Check sheet for the drawn part. Datum: minimum x, y, z corner. Units: mm. A direction names the side the tool comes from. Give positions to 0.01 mm unless a question says otherwise; leave off trailing zeros. Order: outer loops, then holes, each group sorted by start corner. A loop starts at its lowest first (then second) coordinate and runs counter-clockwise, first axis right, second up.
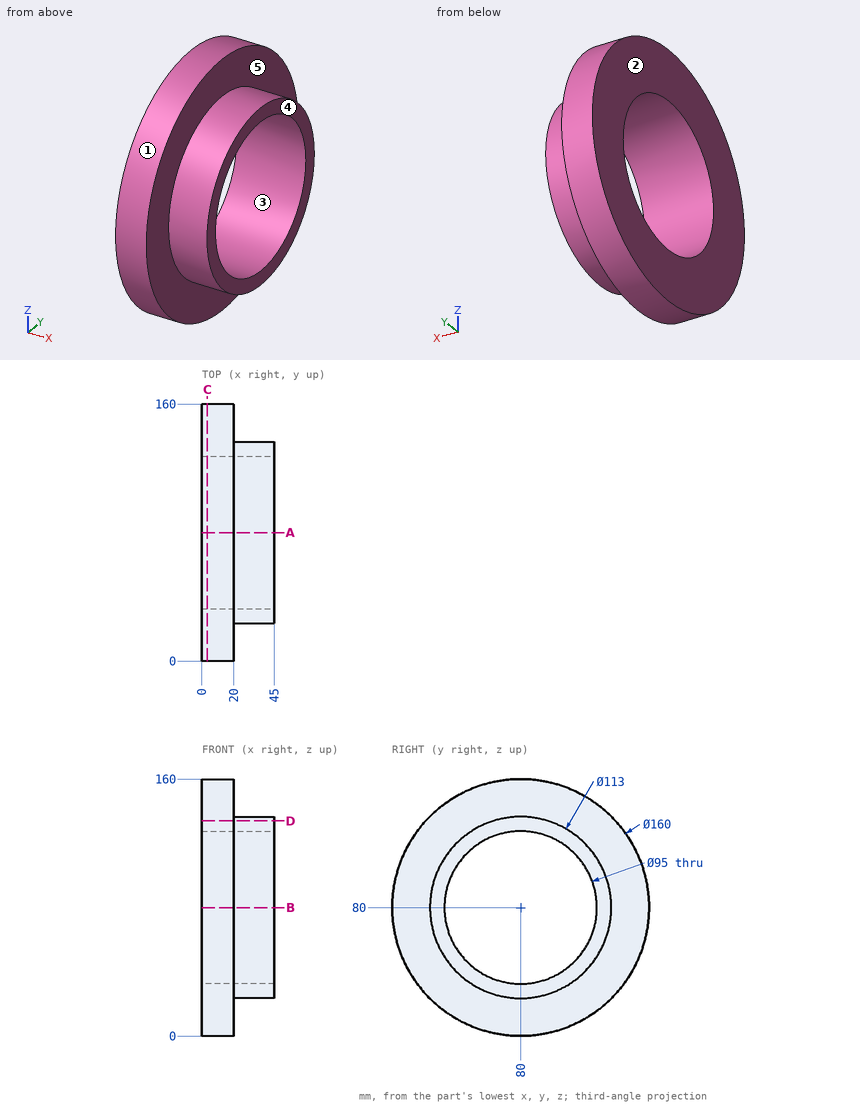
Item 1: Sectioned sample at D-D (z = 134). Enter the section's corners in (x, y), and give its area (3 significant figures).
Reported:
outline: (0, 20.97) - (20, 20.97) - (20, 63.38) - (45, 63.38) - (45, 96.62) - (20, 96.62) - (20, 139.03) - (0, 139.03) - close
area: 3,190 mm2
Item 2: Gauge pin test, flat ends, axial feed: pin 1 (4 mm diameter, centred on x = 33.5, z = 51.5, fed in from +Y); pin 2 (12 mm diameter, centred on y = 129.5, z = 111, fed in from +X); pin 3 (8 mm diameter, centred on x = 30, y = 90.5, fed in from +Z); pin 4 (5 mm diameter, centred on x = 15, y = 63, fed in from -Z). Record the tip position at first contact, or that the pin passes through.
Reported:
pin 1: stops at y = 129.9
pin 2: stops at x = 45
pin 3: stops at z = 136.12
pin 4: stops at z = 1.33
Item 3: Scan lines: L1, parallel to Y at x = 12.5, z = 80; L2, parallel to Y at x = 26, z = 80; L3, parallel to X at y = 57.5, z = 136.5. Record each from-to range of solid material in increasing order.
Reported:
L1: y = 0 to 32.5, 127.5 to 160
L2: y = 23.5 to 32.5, 127.5 to 136.5
L3: x = 0 to 20
Item 4: Set-up check for the marked faces 4 and 5: record each of +Z, -Z, +X, -X, +Y, -Y from which the full face is reachable in a straight line by a thin tool's end or side.
Reported:
face 4: +Z, -Z, +X, +Y, -Y
face 5: +X
Item 5: Draft check along Y on the marked faces 1, 2 and 3. Enter one of: released by +Y, released by -Y, zero draft, split by the parting line, or undercut.
Reported:
face 1: split by the parting line
face 2: zero draft
face 3: undercut
Item 6: Sectioned sample at A-A (y = 80). Enter the section's corners in (x, z), and give its area (3 significant figures).
Reported:
outline: (0, 0) - (20, 0) - (20, 23.5) - (45, 23.5) - (45, 32.5) - (0, 32.5) - close; (0, 127.5) - (45, 127.5) - (45, 136.5) - (20, 136.5) - (20, 160) - (0, 160) - close
area: 1,750 mm2
Item 7: Sectioned sample at C-C (x = 3.5). Enter the section's corners in (y, z), and give its area (3 significant figures).
Reported:
outline: circle Ø160 at (80, 80); hole circle Ø95 at (80, 80)
area: 13,000 mm2
